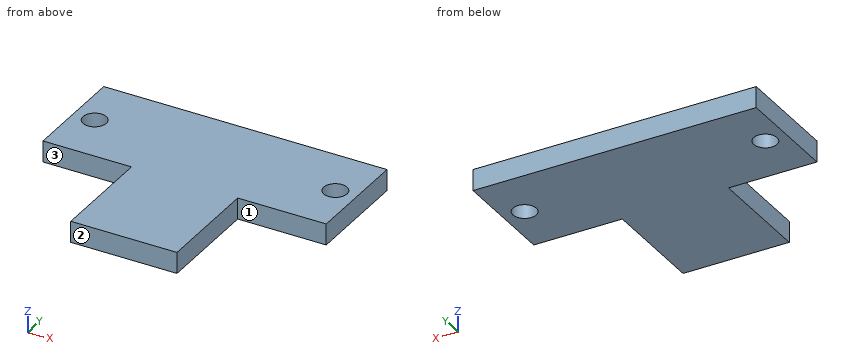
```python
from build123d import *

# Parameters (mm, degrees)
ESQUISSE1_R        = 1.65
BOSS_EXTRU_1_DEPTH = 3


with BuildPart() as part:
    # Esquisse1 → Boss.-Extru.1 (new body)
    with BuildSketch(Plane.XY):
        Polygon((-7.5, -7.5), (-7.5, -22.5), (7.5, -22.5), (7.5, -7.5), (20, -7.5), (20, 7.5), (-20, 7.5), (-20, -7.5), align=None)
        with Locations((-17, 0)):
            Circle(ESQUISSE1_R, mode=Mode.SUBTRACT)
        with Locations((17, 0)):
            Circle(ESQUISSE1_R, mode=Mode.SUBTRACT)
    extrude(amount=-BOSS_EXTRU_1_DEPTH)


solid = part.part
```
For this review, take the finished solid that the model builds, in its own axes (mm). Face numbers are marked on the shaded views. A direction names the side the tool comes from. Give positions to 0.01 mm unless a question says otherwise; leave off trailing zeros. Loops run counter-clockwise (first coordinate to the right, second up) from the corner with the lowest first, then second, coordinate; pieces in that order, holes last. Notation, with made-up numbers: M -16.75,-27 L -5.75,-27 A15 cw -5.75,-6 Z; hole C 66,12 d11. An arc over 180 degrees is marked long. One line per item, written item: value. Start each with the question number.
Q1. Machinability: for the marked faces 1, 2 and 3, which of the approach directions +Z, -Z, +X, -X, +Y, -Y give a long, thin tool a straight path to every point of the face, cutting with its end or side? Answer none if there is none.
Q2. Add section C-C (z = -1.3). Give the boundary of the cut face in (x, y).
Q3. For L1, parallel to Y at x = 17, z = -1.35; L2, parallel to X at y = -1, z = -0.95; L3, parallel to X at y = -8.75, z = -1.35, list the stretches that pass through material, from the lowest coordinate up.
Q4. Add section D-D (y = -12.75). Give the boundary of the cut face in (x, z).
Q5. Add section B-B (y = 0). Give the boundary of the cut face in (x, z).
Q6. Clearance check with flat-ended pins moving along their axes: pin 1 Ø0.9 at (y, z) = (-18.5, -1.5) entering from -X; pin 2 Ø1.5 at (y, z) = (-18, -1) entering from +X; pin 3 Ø0.9 at (x, z) = (-14, -2) entering from -Y. State where each tip first meets the part, or that it passes through.
Q7. Add section A-A (x = 17). Give the boundary of the cut face in (y, z).
Reply:
1. face 1: +Z, -Z, +X, -Y
1. face 2: +Z, -Z, +X, -X, -Y
1. face 3: +Z, -Z, -X, -Y
2. outline: M -20,-7.5 L -7.5,-7.5 L -7.5,-22.5 L 7.5,-22.5 L 7.5,-7.5 L 20,-7.5 L 20,7.5 L -20,7.5 Z; hole C -17,0 d3.3; hole C 17,0 d3.3
3. L1: -7.5 to -1.65, 1.65 to 7.5
3. L2: -20 to -18.31, -15.69 to 15.69, 18.31 to 20
3. L3: -7.5 to 7.5
4. outline: M -7.5,-3 L 7.5,-3 L 7.5,0 L -7.5,0 Z
5. outline: M -20,-3 L -18.65,-3 L -18.65,0 L -20,0 Z; M -15.35,-3 L 15.35,-3 L 15.35,0 L -15.35,0 Z; M 18.65,-3 L 20,-3 L 20,0 L 18.65,0 Z
6. pin 1: x = -7.5
6. pin 2: x = 7.5
6. pin 3: y = -7.5
7. outline: M -7.5,-3 L -1.65,-3 L -1.65,0 L -7.5,0 Z; M 1.65,-3 L 7.5,-3 L 7.5,0 L 1.65,0 Z
